For this review, take the finished solid that the model builds, in its own axes (mm). Face numbers are marked on the shaded views. A direction names the side the tool comes from. Coordinates: 2 decimals unless noted, no trailing zeros. Loops run counter-clockwise (first coordinate to the right, second up) from the corner with the lowest first, then second, coordinate; pieces in that order, holes last.
1. Clearance check with flat-ended pins moving along their axes: P1, Ø8.5, axis at y = 1, z = 3, coming from the -X side; P2, Ø2.5, axis at y = 1, z = 13, coming from the +X side; P3, Ø1.5, axis at x = 1, y = -2, coming from the -Z side. State where each tip first meets the part, or that it passes through.
2. Mouldability with a two-part tool opening along Y and no side actions: class the marked faces 1, 2, 3 and 4 as pulls with the +Y half, pulls with the -Y half, needs draft (parallel to the pull), parting line crosses it, or undercut.
3. Machinability: for the marked faces 5, 6 and 7, which of the approach directions +Z, -Z, +X, -X, +Y, -Y give a long, thin tool a straight path to every point of the face, cutting with its end or side? Answer none if there is none.
4. To check wall thickness, follow probe 1 along Y at (x, z) = (0.7, 0); probe 2 along Y at (x, z) = (3.4, 0); probe 3 along Z at (x, y) = (-0.5, -1). State the ranges of each line that lie inside material, in increasing order.
5. Take a section at A-A, the plane z = -14.5. State the section outline as (x, y) points, then the cut area to 3 significant figures.
6. Take a section at B-B, the plane x = -2. State the section outline as (y, z) points.
7. Take a section at C-C, the plane y = 0. Count the separate pieces of the cut face and the enclosed holes in it, then the cut area to 3 significant figures.
```python
from build123d import *

# Parameters (mm, degrees)
SKETCH_1_W = 8
SKETCH_1_H = 19.5


with BuildPart() as part:
    # ｽｹｯﾁ1 → 回転1 (revolve)
    with BuildSketch(Plane.XY, mode=Mode.PRIVATE) as revolve_1_sk:
        with Locations((0, 9.75)):
            Rectangle(SKETCH_1_W, SKETCH_1_H)
    revolve(revolve_1_sk.sketch.rotate(Axis((4, 0, 0), (-1, 0, 0)), 270), axis=Axis((4, 0, 0), (-1, 0, 0)))

    # ｽｹｯﾁ2 → ｶｯﾄ - 回転1 (revolve, cut)
    with BuildSketch(Plane.XY, mode=Mode.PRIVATE) as cut_revolve_1_sk:
        Polygon((-4, 0), (-4, 8.5), (2, 8.5), (2, 6.5), (4, 6.5), (4, 0), align=None)
    revolve(cut_revolve_1_sk.sketch.rotate(Axis((4, 0, 0), (-1, 0, 0)), 270), axis=Axis((4, 0, 0), (-1, 0, 0)), mode=Mode.SUBTRACT)

    # ｽｹｯﾁ3 → ｶｯﾄ - 回転2 (revolve, cut)
    with BuildSketch(Plane.XY, mode=Mode.PRIVATE) as cut_revolve_2_sk:
        Polygon((-4, 14.5), (-4, 17), (-3.567, 16.567), (-0.833, 16.567), (-0.4, 17), (-0.4, 18.5), (4, 18.5), (4, 14.5), align=None)
    revolve(cut_revolve_2_sk.sketch.rotate(Axis((4, 14.5, 0), (-1, 0, 0)), 270), axis=Axis((4, 14.5, 0), (-1, 0, 0)), mode=Mode.SUBTRACT)

    # ｽｹｯﾁ4 → ｶｯﾄ - 回転3 (revolve, cut)
    with BuildSketch(Plane.XY.offset(14.5), mode=Mode.PRIVATE) as cut_revolve_3_sk:
        Polygon((-4, 0), (-4, 2.5), (-3.567, 2.067), (-0.833, 2.067), (-0.4, 2.5), (-0.4, 4), (4, 4), (4, 0), align=None)
    revolve(cut_revolve_3_sk.sketch.rotate(Axis((4, 0, 14.5), (-1, 0, 0)), 270), axis=Axis((4, 0, 14.5), (-1, 0, 0)), mode=Mode.SUBTRACT)

    # ｽｹｯﾁ5 → ｶｯﾄ - 回転4 (revolve, cut)
    with BuildSketch(Plane.XY, mode=Mode.PRIVATE) as cut_revolve_4_sk:
        Polygon((-4, -14.5), (-4, -12), (-3.567, -12.433), (-0.833, -12.433), (-0.4, -12), (-0.4, -10.5), (4, -10.5), (4, -14.5), align=None)
    revolve(cut_revolve_4_sk.sketch.rotate(Axis((4, -14.5, 0), (-1, 0, 0)), 270), axis=Axis((4, -14.5, 0), (-1, 0, 0)), mode=Mode.SUBTRACT)

    # ｽｹｯﾁ6 → ｶｯﾄ - 回転5 (revolve, cut)
    with BuildSketch(Plane.XY.offset(-14.5), mode=Mode.PRIVATE) as cut_revolve_5_sk:
        Polygon((-4, 0), (-4, 2.5), (-3.567, 2.067), (-0.833, 2.067), (-0.4, 2.5), (-0.4, 4), (4, 4), (4, 0), align=None)
    revolve(cut_revolve_5_sk.sketch.rotate(Axis((4, 0, -14.5), (-1, 0, 0)), 270), axis=Axis((4, 0, -14.5), (-1, 0, 0)), mode=Mode.SUBTRACT)


solid = part.part
```
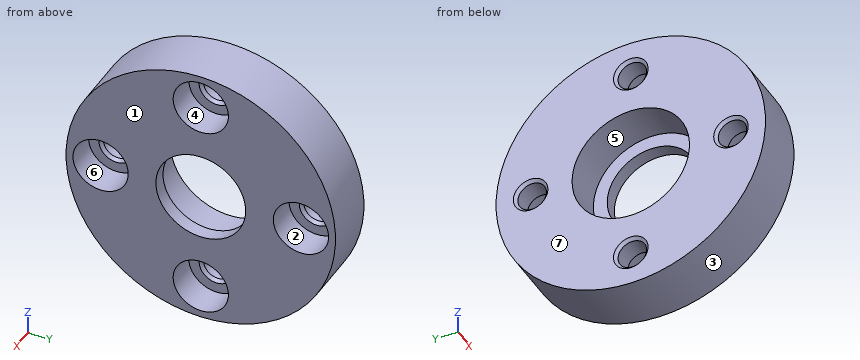
Results list:
1. P1: stops at x = 2
1. P2: stops at x = -0.4
1. P3: stops at z = -19.46
2. face 1: needs draft
2. face 2: undercut
2. face 3: parting line crosses it
2. face 4: undercut
3. face 5: -X
3. face 6: +X
3. face 7: +Z, -Z, -X, +Y, -Y
4. probe 1: y = -19.5 to -18.5, -10.5 to -8.5, 8.5 to 10.5, 18.5 to 19.5
4. probe 2: y = -19.5 to -18.5, -10.5 to -6.5, 6.5 to 10.5, 18.5 to 19.5
4. probe 3: z = -19.47 to -16.68, -12.32 to -8.44, 8.44 to 12.32, 16.68 to 19.47
5. outline: (-4, -13.04) - (4, -13.04) - (4, -4) - (-0.4, -4) - (-0.4, -2.5) - (-0.83, -2.07) - (-3.57, -2.07) - (-4, -2.5) - close; (-4, 2.5) - (-3.57, 2.07) - (-0.83, 2.07) - (-0.4, 2.5) - (-0.4, 4) - (4, 4) - (4, 13.04) - (-4, 13.04) - close
5. area: 158 mm2
6. outline: circle Ø39 at (0, 0); hole circle Ø4.13 at (-14.5, 0); hole circle Ø17 at (0, 0); hole circle Ø4.13 at (0, -14.5); hole circle Ø4.13 at (0, 14.5); hole circle Ø4.13 at (14.5, 0)
7. separate pieces: 4
7. enclosed holes: 0
7. area: 83.1 mm2
